Part model, mm, in its own coordinate system. Face numbers are marked on the shaded views. A direction names the side the tool comes from. Round coordinates to 2 decimals unless told otherwise and drop trailing zeros. Loops run counter-clockwise (first coordinate to the right, second up) from the corner with the lowest first, then second, coordinate; pieces in that order, holes last. Notation, with made-up numbers: (-34.5, 69) -> (-5.5, 69) arc R13 cw to (-5.5, 82) -> close; hole circle Ø7 at (1, 57). An arc over 180 degrees is marked (long way). Use a Markdown table: item, result. Add a question column.
Item 1: Which spindle directions (+Z, -Z, +X, -X, +Y, -Y) get a long thin tool onto all of the face, cutting with end or side? Do the marked faces 1, 2 and 3. Say none if no direction does.
Item 2: Cut at D-D, the plane y = 38. List the corners of the cut face in (x, z), plus the area to 3 significant figures.
Item 3: Cut at B-B, the plane y = 114. List the corners of the cut face in (x, z), plus the area to 3 significant figures.
Item 4: Cut at A-A, the plane x = 69. List the corners of the cut face in (y, z).
Item 5: Flat gauge pins, fed straight in: pin 1 (1.5 mm diameter, centred on x = 85, z = 24, fed in from -Y); pin 2 (8 mm diameter, centred on y = 44, z = 18, fed in from +X); pin 3 (1.5 mm diameter, centred on x = 67, z = -34, fed in from +Y). Where does each tip first touch, or does it go through?
Item 6: Two-plate mould, pull along X, no slides. Class the marked faces 4, 5, 6 and 7: pulls with the +X half, pulls with the -X half, needs draft (parallel to the pull), parting line crosses it, or undercut.
Item 7: Probe line 1 (Y direction, x = 100, z = 0); line 2 (X direction, y = 69, z = -15.5); line 3 (Z direction, x = 42, y = 71.5). List the from-to ranges inside material, lowest first. Write a range as [from, to].
Item 8: Cut at C-C, the plane z = 10.5. List the corners of the cut face in (x, y), plus the area to 3 significant figures.
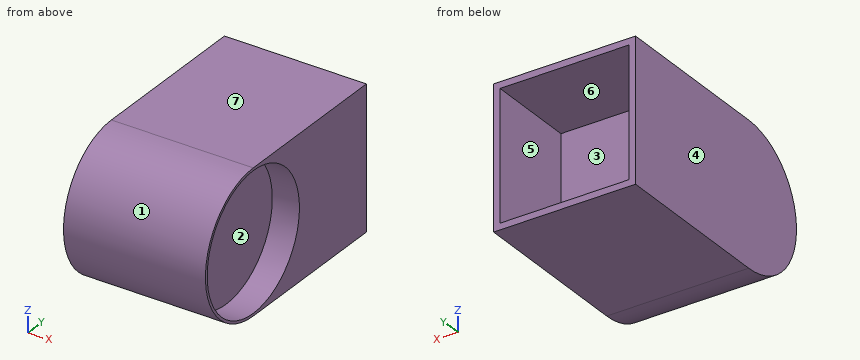
```python
from build123d import *

# Parameters (mm, degrees)
BOSS_EXTRUDE1_DEPTH = 110
SKETCH2_W           = 100
SKETCH2_H           = 100
CUT_EXTRUDE1_DEPTH  = 70
SKETCH3_R           = 53
CUT_EXTRUDE2_DEPTH  = 21


with BuildPart() as part:
    # Sketch1 → Boss-Extrude1 (new body)
    with BuildSketch(Plane(origin=(0, 0, 0), x_dir=(0, 0, -1), z_dir=(1, 0, 0))):
        with BuildLine():
            Line((55, 129.977668722), (55, -2.75e-07))
            ThreePointArc((55, -2.75e-07), (-2.948e-06, -55), (-55, 5.622e-06))
            Line((-55, 5.622e-06), (-55, 129.977668722))
            Line((-55, 129.977668722), (55, 129.977668722))
        make_face()
    extrude(amount=BOSS_EXTRUDE1_DEPTH)

    # Sketch2 → Cut-Extrude1 (cut)
    with BuildSketch(Plane(origin=(0, 129.977668722, 0), x_dir=(1, 0, 0), z_dir=(0, 1, 0))):
        with Locations((55, 0)):
            Rectangle(SKETCH2_W, SKETCH2_H)
    extrude(amount=-CUT_EXTRUDE1_DEPTH, mode=Mode.SUBTRACT)

    # Sketch3 → Cut-Extrude2 (cut)
    with BuildSketch(Plane(origin=(110, 0, 0), x_dir=(0, 0, -1), z_dir=(1, 0, 0))):
        Circle(SKETCH3_R)
    extrude(amount=-CUT_EXTRUDE2_DEPTH, mode=Mode.SUBTRACT)


solid = part.part
```
A:
| question | item | result |
|---|---|---|
| 1 | face 1 | +X, -X, -Y |
| 1 | face 2 | +X |
| 1 | face 3 | +Y |
| 2 | outline | (0, -55) -> (110, -55) -> (110, -36.95) -> (89, -36.95) -> (89, 36.95) -> (110, 36.95) -> (110, 55) -> (0, 55) -> close |
| 2 | area | 10,500 mm^2 |
| 3 | outline | (0, -55) -> (110, -55) -> (110, 55) -> (0, 55) -> close; hole (5, -50) -> (105, -50) -> (105, 50) -> (5, 50) -> close |
| 3 | area | 2,100 mm^2 |
| 4 | outline | (0, -55) -> (129.98, -55) -> (129.98, -50) -> (59.98, -50) -> (59.98, 50) -> (129.98, 50) -> (129.98, 55) -> (0, 55) arc R55 ccw to start |
| 5 | pin 1 | stops at y = -49.84 |
| 5 | pin 2 | stops at x = 89 |
| 5 | pin 3 | stops at y = 59.98 |
| 6 | face 4 | pulls with the -X half |
| 6 | face 5 | undercut |
| 6 | face 6 | undercut |
| 6 | face 7 | needs draft |
| 7 | line 1 | y = [-55, -53], [53, 59.98] |
| 7 | line 2 | x = [0, 5], [105, 110] |
| 7 | line 3 | z = [-55, -50], [50, 55] |
| 8 | outline | (0, -53.99) -> (110, -53.99) -> (110, -51.95) -> (89, -51.95) -> (89, 51.95) -> (110, 51.95) -> (110, 129.98) -> (105, 129.98) -> (105, 59.98) -> (5, 59.98) -> (5, 129.98) -> (0, 129.98) -> close |
| 8 | area | 11,100 mm^2 |
